Part model, mm, in its own coordinate system. A direction names the side the tool comes from. Coordinates: 2 decimals unless noted, no trailing zeros. Write each loop counter-clockwise with the first axis right and the second up, starting at its lowest first coordinate (ties: lowest second). Pieces come first, ordered by that corner, then holes. Notation, with made-up numbers: (84.25, 76) -> (114.25, 76) arc R26 cw to (114.25, 104) -> close; hole circle Ø1 at (18, 30.5). An arc over 180 degrees is marked (long way). Write item = value, one per line.
from build123d import *

# Parameters (mm, degrees)
SKETCH1_W            = 133
SKETCH1_H            = 133
BOSS_EXTRUDE2_DEPTH  = 136
SKETCH2_W            = 133
SKETCH2_H            = 118
CUT_EXTRUDE1_DEPTH   = 136
BOSS_EXTRUDE3_DEPTH  = 10.5
SKETCH5_W            = 21
SKETCH5_H            = 3
BOSS_EXTRUDE4_DEPTH  = 23.5
SKETCH6_W            = 42
SKETCH6_H            = 17.2
CUT_EXTRUDE2_DEPTH   = 3
BOSS_EXTRUDE5_DEPTH  = 10.5
SKETCH8_W            = 21
SKETCH8_H            = 3
BOSS_EXTRUDE6_DEPTH  = 23.5
SKETCH9_W            = 42
SKETCH9_H            = 17.2
CUT_EXTRUDE3_DEPTH   = 3
SKETCH10_W           = 19.261488562
SKETCH10_H           = 133
BOSS_EXTRUDE7_DEPTH  = 5
SKETCH11_W           = 18.43727499
SKETCH11_H           = 133
BOSS_EXTRUDE8_DEPTH  = 5
SKETCH12_W           = 18.849381776
SKETCH12_H           = 146
BOSS_EXTRUDE9_DEPTH  = 12
SKETCH14_W           = 18.849381776
SKETCH14_H           = 146
BOSS_EXTRUDE10_DEPTH = 12
SKETCH17_R           = 1
CUT_EXTRUDE4_DEPTH   = 222.251553667
SKETCH18_W           = 133
SKETCH18_H           = 136
CUT_EXTRUDE5_DEPTH   = 170
SKETCH20_R           = 2.5
CUT_EXTRUDE6_DEPTH   = 10
SKETCH22_R           = 2.5
CUT_EXTRUDE8_DEPTH   = 170
SKETCH24_R           = 2.5
CUT_EXTRUDE9_DEPTH   = 170
SKETCH26_R           = 2.474722671
CUT_EXTRUDE10_DEPTH  = 177
SKETCH27_R           = 2.5
CUT_EXTRUDE11_DEPTH  = 177
SKETCH29_R           = 2.5
CUT_EXTRUDE12_DEPTH  = 177
SKETCH30_R           = 2.5
CUT_EXTRUDE13_DEPTH  = 178
SKETCH31_R           = 2.5
CUT_EXTRUDE14_DEPTH  = 178
SKETCH32_R           = 2.474722671
SKETCH32_R_2         = 2.5
BOSS_EXTRUDE11_DEPTH = 5
SKETCH33_R           = 2.5
BOSS_EXTRUDE12_DEPTH = 5


with BuildPart() as part:
    # Sketch1 → Boss-Extrude2 (new body)
    with BuildSketch(Plane(origin=(0, 0, 0), x_dir=(1, 0, 0), z_dir=(0, 1, 0))):
        Rectangle(SKETCH1_W, SKETCH1_H)
    extrude(amount=BOSS_EXTRUDE2_DEPTH)

    # Sketch2 → Cut-Extrude1 (cut)
    with BuildSketch(Plane.XY.offset(66.5)):
        with Locations((0, 68)):
            Rectangle(SKETCH2_W, SKETCH2_H)
    extrude(amount=-CUT_EXTRUDE1_DEPTH, mode=Mode.SUBTRACT)


with BuildPart() as cut_extrude1_piece_1:
    # of the separate pieces the step leaves, piece 1, a body of its own (cut_extrude1_pieces)
    add(part.part.solids().sort_by_distance((-66.5, 0, 66.5))[0])

    # Sketch4 → Boss-Extrude3 (add)
    with BuildSketch(Plane(origin=(0, 9, 0), x_dir=(1, 0, 0), z_dir=(0, 1, 0))):
        Polygon((22.75, -22.75), (43.75, -22.75), (46.25, -22.75), (46.25, -20.25), (20.25, -20.25), (20.25, -46.25), (46.25, -46.25), (46.25, -43.75), (43.75, -43.75), (22.75, -43.75), align=None)
        Polygon((22.75, 43.75), (43.75, 43.75), (46.25, 43.75), (46.25, 46.25), (20.25, 46.25), (20.25, 20.25), (46.25, 20.25), (46.25, 22.75), (43.75, 22.75), (22.75, 22.75), align=None)
    extrude(amount=BOSS_EXTRUDE3_DEPTH)

    # Sketch5 → Boss-Extrude4 (add)
    with BuildSketch(Plane(origin=(22.75, 0, 0), x_dir=(0, 0, -1), z_dir=(1, 0, 0))):
        with Locations((-33.25, 18)):
            Rectangle(SKETCH5_W, SKETCH5_H)
        with Locations((33.25, 18)):
            Rectangle(SKETCH5_W, SKETCH5_H)
    extrude(amount=BOSS_EXTRUDE4_DEPTH)

    # Sketch6 → Cut-Extrude2 (cut)
    with BuildSketch(Plane(origin=(0, 19.5, 0), x_dir=(1, 0, 0), z_dir=(0, 1, 0))):
        with Locations((46.25, -33.25)):
            Rectangle(SKETCH6_W, SKETCH6_H)
        with Locations((46.25, 33.25)):
            Rectangle(SKETCH6_W, SKETCH6_H)
    extrude(amount=-CUT_EXTRUDE2_DEPTH, mode=Mode.SUBTRACT)

    # Sketch10 → Boss-Extrude7 (add)
    with BuildSketch(Plane.XZ):
        Rectangle(SKETCH10_W, SKETCH10_H)
    extrude(amount=BOSS_EXTRUDE7_DEPTH)



with BuildPart() as cut_extrude1_piece_2:
    # of the separate pieces the step leaves, piece 2, a body of its own (cut_extrude1_pieces)
    add(part.part.solids().sort_by_distance((66.5, 127, 66.5))[0])

    # Sketch7 → Boss-Extrude5 (add)
    with BuildSketch(Plane.XZ.offset(-127)):
        Polygon((-43.75, 43.75), (-22.75, 43.75), (-22.75, 22.75), (-43.75, 22.75), (-46.25, 22.75), (-46.25, 20.25), (-20.25, 20.25), (-20.25, 46.25), (-46.25, 46.25), (-46.25, 43.75), align=None)
        Polygon((-43.75, -22.75), (-22.75, -22.75), (-22.75, -43.75), (-43.75, -43.75), (-46.25, -43.75), (-46.25, -46.25), (-20.25, -46.25), (-20.25, -20.25), (-46.25, -20.25), (-46.25, -22.75), align=None)
    extrude(amount=BOSS_EXTRUDE5_DEPTH)

    # Sketch8 → Boss-Extrude6 (add)
    with BuildSketch(Plane.ZY.offset(22.75)):
        with Locations((33.25, 118)):
            Rectangle(SKETCH8_W, SKETCH8_H)
        with Locations((-33.25, 118)):
            Rectangle(SKETCH8_W, SKETCH8_H)
    extrude(amount=BOSS_EXTRUDE6_DEPTH)

    # Sketch9 → Cut-Extrude3 (cut)
    with BuildSketch(Plane.XZ.offset(-116.5)):
        with Locations((-46.25, 33.25)):
            Rectangle(SKETCH9_W, SKETCH9_H)
        with Locations((-46.25, -33.25)):
            Rectangle(SKETCH9_W, SKETCH9_H)
    extrude(amount=-CUT_EXTRUDE3_DEPTH, mode=Mode.SUBTRACT)

    # Sketch11 → Boss-Extrude8 (add)
    with BuildSketch(Plane(origin=(0, 136, 0), x_dir=(1, 0, 0), z_dir=(0, 1, 0))):
        Rectangle(SKETCH11_W, SKETCH11_H)
    extrude(amount=BOSS_EXTRUDE8_DEPTH)


with BuildPart() as cut_extrude1_piece_1_1:
    add(cut_extrude1_piece_1.part)

    add(cut_extrude1_piece_2.part)  # Boss-Extrude9 merges Cut-Extrude1 piece 2
    # Sketch12 → Boss-Extrude9 (add)
    with BuildSketch(Plane(origin=(0, 0, -66.5), x_dir=(-1, 0, 0), z_dir=(0, 0, -1))):
        with Locations((-0.206053393, 68)):
            Rectangle(SKETCH12_W, SKETCH12_H)
    extrude(amount=BOSS_EXTRUDE9_DEPTH)

    # Sketch14 → Boss-Extrude10 (add)
    with BuildSketch(Plane.XY.offset(66.5)):
        with Locations((0.206053393, 68)):
            Rectangle(SKETCH14_W, SKETCH14_H)
    extrude(amount=BOSS_EXTRUDE10_DEPTH)

    # Sketch17 → Cut-Extrude4 (cut, through all)
    with BuildSketch(Plane.XY.offset(78.5)):
        with Locations((0.206053393, 68)):
            Circle(SKETCH17_R)
    extrude(amount=-CUT_EXTRUDE4_DEPTH, mode=Mode.SUBTRACT)

    # Sketch18 → Cut-Extrude5 (cut)
    with BuildSketch(Plane.ZY.offset(66.5)):
        with Locations((0, 68)):
            Rectangle(SKETCH18_W, SKETCH18_H)
    extrude(amount=-CUT_EXTRUDE5_DEPTH, mode=Mode.SUBTRACT)

    # Sketch20 → Cut-Extrude6 (cut)
    with BuildSketch(Plane(origin=(0, 0, 0), x_dir=(1, 0, 0), z_dir=(0, 1, 0))):
        with Locations(Location((0, 0, 0), (0, 0, 270))):
            Circle(SKETCH20_R)
    extrude(amount=-CUT_EXTRUDE6_DEPTH, mode=Mode.SUBTRACT)

    # Sketch22 → Cut-Extrude8 (cut)
    with BuildSketch(Plane(origin=(0, 0, 0), x_dir=(1, 0, 0), z_dir=(0, 1, 0))):
        with Locations(Location((0, 0, 0), (0, 0, 270))):
            Circle(SKETCH22_R)
    extrude(amount=CUT_EXTRUDE8_DEPTH, mode=Mode.SUBTRACT)

    # Sketch24 → Cut-Extrude9 (cut)
    with BuildSketch(Plane(origin=(0, 0, 0), x_dir=(1, 0, 0), z_dir=(0, 1, 0))):
        with Locations(Location((0, 59.159797643, 0), (0, 0, 270))):
            Circle(SKETCH24_R)
    extrude(amount=-CUT_EXTRUDE9_DEPTH, mode=Mode.SUBTRACT)

    # Sketch26 → Cut-Extrude10 (cut)
    with BuildSketch(Plane(origin=(0, 9, 0), x_dir=(1, 0, 0), z_dir=(0, 1, 0))):
        with Locations(Location((0, 59.159797643, 0), (0, 0, 90))):
            Circle(SKETCH26_R)
    extrude(amount=CUT_EXTRUDE10_DEPTH, mode=Mode.SUBTRACT)

    # Sketch27 → Cut-Extrude11 (cut)
    with BuildSketch(Plane(origin=(0, 0, 0), x_dir=(1, 0, 0), z_dir=(0, 1, 0))):
        with Locations(Location((0, -59.499471122, 0), (0, 0, 270))):
            Circle(SKETCH27_R)
    extrude(amount=-CUT_EXTRUDE11_DEPTH, mode=Mode.SUBTRACT)

    # Sketch29 → Cut-Extrude12 (cut)
    with BuildSketch(Plane.XZ.offset(5)):
        with Locations(Location((0, 59.499471122, 0), (0, 0, 90))):
            Circle(SKETCH29_R)
    extrude(amount=-CUT_EXTRUDE12_DEPTH, mode=Mode.SUBTRACT)

    # Sketch30 → Cut-Extrude13 (cut)
    with BuildSketch(Plane(origin=(0, 141, 0), x_dir=(1, 0, 0), z_dir=(0, 1, 0))):
        with Locations(Location((0, 37.126366322, 0), (0, 0, 270))):
            Circle(SKETCH30_R)
    extrude(amount=-CUT_EXTRUDE13_DEPTH, mode=Mode.SUBTRACT)

    # Sketch31 → Cut-Extrude14 (cut)
    with BuildSketch(Plane(origin=(0, 141, 0), x_dir=(1, 0, 0), z_dir=(0, 1, 0))):
        with Locations(Location((0, -34.245307912, 0), (0, 0, 270))):
            Circle(SKETCH31_R)
    extrude(amount=-CUT_EXTRUDE14_DEPTH, mode=Mode.SUBTRACT)

    # Sketch32 → Boss-Extrude11 (add)
    with BuildSketch(Plane(origin=(0, 141, 0), x_dir=(1, 0, 0), z_dir=(0, 1, 0))):
        with Locations((0, 59.159797643)):
            Circle(SKETCH32_R)
        with Locations(Location((0, -59.499471122, 0), (0, 0, 270))):
            Circle(SKETCH32_R_2)
    extrude(amount=-BOSS_EXTRUDE11_DEPTH)

    # Sketch33 → Boss-Extrude12 (add)
    with BuildSketch(Plane.XZ.offset(5)):
        with Locations((0, -59.159797643)):
            Circle(SKETCH33_R)
        with Locations((0, 59.499471122)):
            Circle(SKETCH33_R)
    extrude(amount=-BOSS_EXTRUDE12_DEPTH)


solid = cut_extrude1_piece_1_1.part
Q1. Probe line 1 (Z direction, x = 5.75, y = 15); line 2 (Y direction, x = -3.5, z = -49.5); line 3 (X direction, y = 68, z = -76). List the from-to ranges inside material, lowest first. Write a range as from..to.
Model answer:
line_1 = -78.5..-66.5, 66.5..78.5
line_2 = -5..0, 136..141
line_3 = -9.22..-0.79, 1.21..9.63
Q2. Pin check, flat tips, straight feed: pin 1 (6.5 mm diameter, centred on x = 0, z = -37.13, fed in from -Y); pin 2 (4 mm diameter, centred on y = 139, z = 30, fed in from +X); pin 3 (0.5 mm diameter, centred on x = -9.5, y = -3.5, fed in from +Z). Stop position of each tip, or through.
Model answer:
pin_1 = -5
pin_2 = 9.22
pin_3 = 66.5
Q3. Saw through at B-B on y = 75. Give the cut face in (x, z), and give its area (3 significant figures).
Model answer:
outline = (-9.22, -78.5) -> (9.63, -78.5) -> (9.63, -66.5) -> (-9.22, -66.5) -> close; (-9.22, 66.5) -> (9.63, 66.5) -> (9.63, 78.5) -> (-9.22, 78.5) -> close
area = 452 mm²
Q4. Mould opens along Y. For faces 4 (the face through (-0.958, -2.465, 36.555)), 5 (the face through (-4, 141, -1)), 6 (the face through (0, 70, 66.5)), 7 (the face through (-4, -5, 1)) say: released by +Y, released by -Y, zero draft, split by the parting line, or undercut.
Model answer:
face_4 = zero draft
face_5 = released by +Y
face_6 = undercut
face_7 = released by -Y
Q5. Which spindle directions (+Z, -Z, +X, -X, +Y, -Y) get a long thin tool onto all of the face, cutting with end or side? Do faces 1 (the face through (-2, 69, 78.5)), 2 (the face through (0, 70, -66.5)), 3 (the face through (9.219, 138, 1)). Say none if no direction does.
Model answer:
face_1 = +Z, +X, -X, +Y, -Y
face_2 = +X, -X
face_3 = +X, +Y
Q6. Saw through at D-D on z = 0. Give the cut face in (x, y), and give its area (3 significant figures).
Model answer:
outline = (-9.63, -5) -> (-2.5, -5) -> (-2.5, 0) -> (-9.63, 0) -> close; (-9.22, 136) -> (-2.5, 136) -> (-2.5, 141) -> (-9.22, 141) -> close; (2.5, -5) -> (9.63, -5) -> (9.63, 0) -> (2.5, 0) -> close; (2.5, 136) -> (9.22, 136) -> (9.22, 141) -> (2.5, 141) -> close
area = 138 mm²
Q7. Saw through at A-A on x = 5.5. Give the cut face in (y, z), and give its area (3 significant figures).
Model answer:
outline = (-5, -78.5) -> (141, -78.5) -> (141, 78.5) -> (-5, 78.5) -> close; hole (0, -66.5) -> (136, -66.5) -> (136, 66.5) -> (0, 66.5) -> close
area = 4,830 mm²
Q8. Saw through at C-C on z = -22.5. Give the cut face in (x, y), and give its area (3 significant figures).
Model answer:
outline = (-9.63, -5) -> (9.63, -5) -> (9.63, 0) -> (-9.63, 0) -> close; (-9.22, 136) -> (9.22, 136) -> (9.22, 141) -> (-9.22, 141) -> close
area = 188 mm²
